The listing builds one solid part. Answer for the finished solid, in the listing's coordinates (mm). Face numbers are marked on the shaded views. A direction names the side the tool comes from. Coordinates: 2 decimals unless noted, no trailing zeros. Loops run counter-clockwise (first coordinate to the right, second up) from the corner with the lowest first, then second, coordinate; pieces in that order, holes last. Notation, with made-up numbers: M -13.75,67.5 L 34.25,67.5 A21 cw 34.25,88.5 Z; hole C 52,-20.5 d3. An arc over 180 degrees is marked long. Answer in a Markdown table with one row per item. Add a question column.
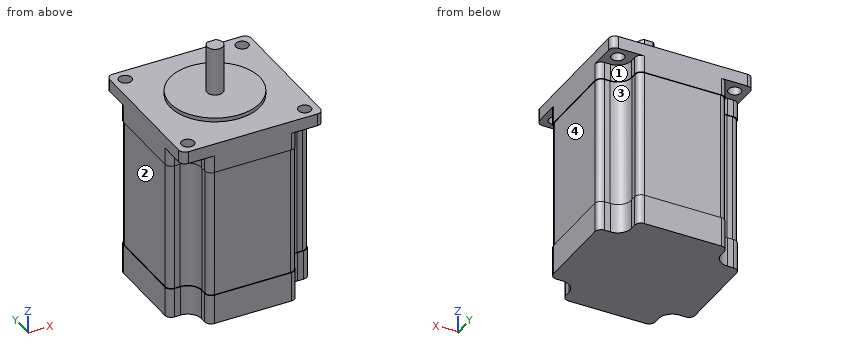
from build123d import *

# Parameters (mm, degrees)
SKETCH1_W           = 57
SKETCH1_H           = 57
SKETCH1_R           = 2.55
BOSS_EXTRUDE1_DEPTH = 5
BOSS_EXTRUDE2_DEPTH = 7
BOSS_EXTRUDE5_DEPTH = 52
BOSS_EXTRUDE6_DEPTH = 12
SKETCH7_R           = 18.05
BOSS_EXTRUDE7_DEPTH = 1.6
SKETCH8_R           = 3.175
BOSS_EXTRUDE8_DEPTH = 21
SKETCH9_W           = 15
SKETCH9_H           = 0.5
CUT_EXTRUDE1_DEPTH  = 3.5
FILLET1_R           = 2.54


with BuildPart() as part:
    # Sketch1 → Boss-Extrude1 (new body)
    with BuildSketch(Plane.XY):
        Rectangle(SKETCH1_W, SKETCH1_H)
        with Locations((-23.5, 23.5)):
            Circle(SKETCH1_R, mode=Mode.SUBTRACT)
        with Locations((23.5, 23.5)):
            Circle(SKETCH1_R, mode=Mode.SUBTRACT)
        with Locations((23.5, -23.5)):
            Circle(SKETCH1_R, mode=Mode.SUBTRACT)
        with Locations((-23.5, -23.5)):
            Circle(SKETCH1_R, mode=Mode.SUBTRACT)
    extrude(amount=-BOSS_EXTRUDE1_DEPTH)

    # Sketch2 → Boss-Extrude2 (add)
    with BuildSketch(Plane(origin=(0, 0, -5), x_dir=(-1, 0, 0), z_dir=(0, 0, -1))):
        with BuildLine():
            Line((-18.05, 23.5), (-18.05, 28.5))
            Line((-18.05, 28.5), (18.05, 28.5))
            Line((18.05, 28.5), (18.05, 23.5))
            ThreePointArc((18.05, 23.5), (19.646268043, 19.646268043), (23.5, 18.05))
            Line((23.5, 18.05), (28.5, 18.05))
            Line((28.5, 18.05), (28.5, -18.05))
            Line((28.5, -18.05), (23.5, -18.05))
            ThreePointArc((23.5, -18.05), (19.646268043, -19.646268043), (18.05, -23.5))
            Line((18.05, -23.5), (18.05, -28.5))
            Line((18.05, -28.5), (-18.05, -28.5))
            Line((-18.05, -28.5), (-18.05, -23.5))
            ThreePointArc((-18.05, -23.5), (-19.646268043, -19.646268043), (-23.5, -18.05))
            Line((-23.5, -18.05), (-28.5, -18.05))
            Line((-28.5, -18.05), (-28.5, 18.05))
            Line((-28.5, 18.05), (-23.5, 18.05))
            ThreePointArc((-23.5, 18.05), (-19.646268043, 19.646268043), (-18.05, 23.5))
        make_face()
    extrude(amount=BOSS_EXTRUDE2_DEPTH)

    # Sketch5 → Boss-Extrude5 (add)
    with BuildSketch(Plane(origin=(0, 0, -12), x_dir=(-1, 0, 0), z_dir=(0, 0, -1))):
        with BuildLine():
            Line((-23.5, 17.796), (-28.246, 17.796))
            Line((-28.246, 17.796), (-28.246, -17.796))
            Line((-28.246, -17.796), (-23.5, -17.796))
            ThreePointArc((-23.5, -17.796), (-19.46666292, -19.46666292), (-17.796, -23.5))
            Line((-17.796, -23.5), (-17.796, -28.246))
            Line((-17.796, -28.246), (17.796, -28.246))
            Line((17.796, -28.246), (17.796, -23.5))
            ThreePointArc((17.796, -23.5), (19.46666292, -19.46666292), (23.5, -17.796))
            Line((23.5, -17.796), (28.246, -17.796))
            Line((28.246, -17.796), (28.246, 17.796))
            Line((28.246, 17.796), (23.5, 17.796))
            ThreePointArc((23.5, 17.796), (19.46666292, 19.46666292), (17.796, 23.5))
            Line((17.796, 23.5), (17.796, 28.246))
            Line((17.796, 28.246), (-17.796, 28.246))
            Line((-17.796, 28.246), (-17.796, 23.5))
            ThreePointArc((-17.796, 23.5), (-19.46666292, 19.46666292), (-23.5, 17.796))
        make_face()
    extrude(amount=BOSS_EXTRUDE5_DEPTH)

    # Sketch6 → Boss-Extrude6 (add)
    with BuildSketch(Plane(origin=(0, 0, -64), x_dir=(-1, 0, 0), z_dir=(0, 0, -1))):
        with BuildLine():
            Line((-23.5, 18.05), (-28.5, 18.05))
            Line((-28.5, 18.05), (-28.5, -18.05))
            Line((-28.5, -18.05), (-23.5, -18.05))
            ThreePointArc((-23.5, -18.05), (-19.646268043, -19.646268043), (-18.05, -23.5))
            Line((-18.05, -23.5), (-18.05, -28.5))
            Line((-18.05, -28.5), (18.05, -28.5))
            Line((18.05, -28.5), (18.05, -23.5))
            ThreePointArc((18.05, -23.5), (19.646268043, -19.646268043), (23.5, -18.05))
            Line((23.5, -18.05), (28.5, -18.05))
            Line((28.5, -18.05), (28.5, 18.05))
            Line((28.5, 18.05), (23.5, 18.05))
            ThreePointArc((23.5, 18.05), (19.646268043, 19.646268043), (18.05, 23.5))
            Line((18.05, 23.5), (18.05, 28.5))
            Line((18.05, 28.5), (-18.05, 28.5))
            Line((-18.05, 28.5), (-18.05, 23.5))
            ThreePointArc((-18.05, 23.5), (-19.646268043, 19.646268043), (-23.5, 18.05))
        make_face()
    extrude(amount=BOSS_EXTRUDE6_DEPTH)

    # Sketch7 → Boss-Extrude7 (add)
    with BuildSketch(Plane.XY):
        with Locations(Location((0, 0, 0), (0, 0, 180))):
            Circle(SKETCH7_R)
    extrude(amount=BOSS_EXTRUDE7_DEPTH)

    # Sketch8 → Boss-Extrude8 (add)
    with BuildSketch(Plane.XY):
        with Locations(Location((0, 0, 0), (0, 0, 180))):
            Circle(SKETCH8_R)
    extrude(amount=BOSS_EXTRUDE8_DEPTH)

    # Sketch9 → Cut-Extrude1 (cut, symmetric)
    with BuildSketch(Plane(origin=(0, 0, 0), x_dir=(0, 0, -1), z_dir=(1, 0, 0))):
        with Locations((-13.5, 2.925)):
            Rectangle(SKETCH9_W, SKETCH9_H)
    extrude(amount=CUT_EXTRUDE1_DEPTH, both=True, mode=Mode.SUBTRACT)

    # Fillet1
    fillet1_edges = [part.edges().sort_by_distance(p)[0] for p in [
        (28.5, 18.05, -70),
        (28.5, -18.05, -70),
        (18.05, -28.5, -70),
        (-18.05, -28.5, -70),
        (-28.5, -18.05, -70),
        (-28.5, 18.05, -70),
        (-18.05, 28.5, -70),
        (18.05, 28.5, -70),
        (28.5, 18.05, -8.5),
        (28.5, -18.05, -8.5),
        (18.05, -28.5, -8.5),
        (-18.05, -28.5, -8.5),
        (-28.5, -18.05, -8.5),
        (-28.5, 18.05, -8.5),
        (-18.05, 28.5, -8.5),
        (18.05, 28.5, -8.5),
        (28.5, -28.5, -2.5),
        (-28.5, -28.5, -2.5),
        (-28.5, 28.5, -2.5),
        (28.5, 28.5, -2.5),
        (28.246, 17.796, -38),
        (28.246, -17.796, -38),
        (17.796, -28.246, -38),
        (-17.796, -28.246, -38),
        (-28.246, -17.796, -38),
        (-28.246, 17.796, -38),
        (-17.796, 28.246, -38),
        (17.796, 28.246, -38),
    ]]
    fillet(fillet1_edges, radius=FILLET1_R)


solid = part.part
(1) Straight lines are drawn through the part: line 1 (Y direction, x = -23.5, z = -1.5); line 2 (X direction, y = -11.5, z = -25); line 3 (Z direction, x = 0, y = -19). For each, find the intervals that lie inside material, in ascending order.
(2) A cutting plane is placed at B-B (x = 0). Give the vertices of the cut face in (y, z) (3 decimals).
(3) A cutting plane is placed at C-C (y = -13). Give the vertices of the cut face in (x, z).
(4) A cutting plane is placed at D-D (z = 14.5). Give the vertices of the cut face in (x, y) (3 decimals), plus the area to 3 significant figures.
(5) A cutting plane is placed at A-A (z = -54.5). Give the vertices of the cut face in (x, y), plus the area to 3 significant figures.
(6) For the marked faces 1, 2, 3 and 4, determine the directions among +Z, -Z, +X, -X, +Y, -Y from which every point of the face is accessible in a straight line to the end or side of a thin tool.
(7) Each of these flat-tipped pins is pushed along its axis until it touches: pin 1 (2.5 mm diameter, centred on y = -24, z = -71.5, fed in from -X); pin 2 (3 mm diameter, centred on x = 20.5, y = 10.5, fed in from +Z); pin 3 (6 mm diameter, centred on x = 18, z = -53, fed in from -Y); pin 4 (4 mm diameter, centred on x = -23.5, y = -23.5, fed in from +Z). Where does it stop, or does it pass through?
Solved:
| question | item | result |
|---|---|---|
| 1 | line 1 | y = -28.5 to -26.05, -20.95 to 20.95, 26.05 to 28.5 |
| 1 | line 2 | x = -28.25 to 28.25 |
| 1 | line 3 | z = -76 to 0 |
| 2 | outline | M -28.5,-76 L 28.5,-76 L 28.5,-64 L 28.246,-64 L 28.246,-12 L 28.5,-12 L 28.5,0 L 18.05,0 L 18.05,1.6 L 3.175,1.6 L 3.175,6 L 2.675,6 L 2.675,21 L -3.175,21 L -3.175,1.6 L -18.05,1.6 L -18.05,0 L -28.5,0 L -28.5,-12 L -28.246,-12 L -28.246,-64 L -28.5,-64 Z |
| 3 | outline | M -28.5,-76 L 28.5,-76 L 28.5,-64 L 28.25,-64 L 28.25,-12 L 28.5,-12 L 28.5,0 L 12.52,0 L 12.52,1.6 L -12.52,1.6 L -12.52,0 L -28.5,0 L -28.5,-12 L -28.25,-12 L -28.25,-64 L -28.5,-64 Z |
| 4 | outline | M -1.71,2.675 A3.175 ccw long 1.71,2.675 Z |
| 4 | area | 30.5 mm² |
| 5 | outline | M -28.25,-15.26 A2.54 ccw -25.71,-17.8 L -23.5,-17.8 A5.7 cw -17.8,-23.5 L -17.8,-25.71 A2.54 ccw -15.26,-28.25 L 15.26,-28.25 A2.54 ccw 17.8,-25.71 L 17.8,-23.5 A5.7 cw 23.5,-17.8 L 25.71,-17.8 A2.54 ccw 28.25,-15.26 L 28.25,15.26 A2.54 ccw 25.71,17.8 L 23.5,17.8 A5.7 cw 17.8,23.5 L 17.8,25.71 A2.54 ccw 15.26,28.25 L -15.26,28.25 A2.54 ccw -17.8,25.71 L -17.8,23.5 A5.7 cw -23.5,17.8 L -25.71,17.8 A2.54 ccw -28.25,15.26 Z |
| 5 | area | 2,770 mm² |
| 6 | face 1 | -Z, +X, +Y |
| 6 | face 2 | -X, +Y, -Y |
| 6 | face 3 | +X, +Y |
| 6 | face 4 | +X, +Y, -Y |
| 7 | pin 1 | stops at x = -18.1 |
| 7 | pin 2 | stops at z = 0 |
| 7 | pin 3 | stops at y = -28.25 |
| 7 | pin 4 | passes through |
